Part model, mm, in its own coordinate system. A direction names the side the tool comes from. Round coordinates to 2 decimals unless told otherwise and drop trailing zeros. Order: outer loops, then holes, each group sorted by start corner. A loop starts at its lowest first (then second) coordinate and runs counter-clockwise, first axis right, second up. Notation, with made-up numbers: M -33.75,20.25 L -0.75,20.25 A23 ccw -0.75,55.25 Z; hole C 63,-32 d7. An arc over 180 degrees is marked long. One line per question, with ' | ' between items.
from build123d import *

# Parameters (mm, degrees)
ESBO_O1_R                = 1.5
ESBO_O1_R_2              = 1.25
RESSALTO_EXTRUS_O1_DEPTH = 5


with BuildPart() as part:
    # Esboço1 → Ressalto-extrusão1 (new body)
    with BuildSketch(Plane(origin=(0, 0, 0), x_dir=(1, 0, 0), z_dir=(0, 1, 0))):
        with BuildLine():
            Line((65, -55), (-65, -55))
            ThreePointArc((-65, -55), (-72.071067812, -52.071067812), (-75, -45))
            Line((-75, -45), (-75, 45))
            ThreePointArc((-75, 45), (-72.071067812, 52.071067812), (-65, 55))
            Line((-65, 55), (65, 55))
            ThreePointArc((65, 55), (72.071067812, 52.071067812), (75, 45))
            Line((75, 45), (75, -45))
            ThreePointArc((75, -45), (72.071067812, -52.071067812), (65, -55))
        make_face()
        with Locations(Location((-40, -50, 0), (0, 0, 270))):
            Circle(ESBO_O1_R, mode=Mode.SUBTRACT)
        with Locations(Location((40, -50, 0), (0, 0, 270))):
            Circle(ESBO_O1_R, mode=Mode.SUBTRACT)
        with Locations(Location((40, 50, 0), (0, 0, 90))):
            Circle(ESBO_O1_R, mode=Mode.SUBTRACT)
        with Locations(Location((-40, 50, 0), (0, 0, 90))):
            Circle(ESBO_O1_R, mode=Mode.SUBTRACT)
        with Locations(Location((17.2, 19.5, 0), (0, 0, 270))):
            Circle(ESBO_O1_R_2, mode=Mode.SUBTRACT)
        with Locations(Location((17.2, -2.5, 0), (0, 0, 270))):
            Circle(ESBO_O1_R_2, mode=Mode.SUBTRACT)
        with Locations(Location((17.2, -24.5, 0), (0, 0, 270))):
            Circle(ESBO_O1_R_2, mode=Mode.SUBTRACT)
        with Locations(Location((-17.2, -24.5, 0), (0, 0, 90))):
            Circle(ESBO_O1_R_2, mode=Mode.SUBTRACT)
        with Locations(Location((-17.2, -2.5, 0), (0, 0, 90))):
            Circle(ESBO_O1_R_2, mode=Mode.SUBTRACT)
        with Locations(Location((-17.2, 19.5, 0), (0, 0, 90))):
            Circle(ESBO_O1_R_2, mode=Mode.SUBTRACT)
        with BuildLine():
            Line((14, 30), (-14, 30))
            ThreePointArc((-14, 30), (-14.707106781, 29.707106781), (-15, 29))
            Line((-15, 29), (-15, -29))
            ThreePointArc((-15, -29), (-14.707106781, -29.707106781), (-14, -30))
            Line((-14, -30), (14, -30))
            ThreePointArc((14, -30), (14.707106781, -29.707106781), (15, -29))
            Line((15, -29), (15, 29))
            ThreePointArc((15, 29), (14.707106781, 29.707106781), (14, 30))
        make_face(mode=Mode.SUBTRACT)
    extrude(amount=RESSALTO_EXTRUS_O1_DEPTH)


solid = part.part
1) Two-plate mould, pull along Z, no slides. Class faces 3 (the face through (39.1, 2.5, 48.8)), 4 (the face through (-16, 0, -1)), 5 (the face through (72.15, 2.46, 51.99)), 6 (the face through (71.99, 2.46, -52.15)): released by +Z, released by -Z, zero draft, split by the parting line, or undercut.
The answers:
face 3: undercut | face 4: zero draft | face 5: released by +Z | face 6: released by -Z
2) Drop flat-ended pins along their axis: pin 1 (2 mm diameter, centred on x = 17.2, z = -19.5, fed in from -Y) (3 decimals); pin 2 (3.5 mm diameter, centred on x = 40, z = -50, fed in from +Y). Give the stop position or say it passes through.
The answers:
pin 1: passes through | pin 2: stops at y = 5
3) Saw through at A-A (z = -10). List the corners of the cut face in (x, y).
The answers:
outline: M -75,0 L -15,0 L -15,5 L -75,5 Z; M 15,0 L 75,0 L 75,5 L 15,5 Z
4) Probe line 1 (Z direction, x = -17.2, y = 1.7); line 2 (X direction, y = 1.35, z = -19.5); line 3 (X direction, y = 1.9, z = -11). List the from-to ranges inside material, lowest first. Write a range as [from, to].
The answers:
line 1: z = [-55, -20.75], [-18.25, 1.25], [3.75, 23.25], [25.75, 55] | line 2: x = [-75, -18.45], [-15.95, -15], [15, 15.95], [18.45, 75] | line 3: x = [-75, -15], [15, 75]
5) Saw through at D-D (x = 7.5). List the corners of the cut face in (y, z).
The answers:
outline: M 0,-55 L 5,-55 L 5,-30 L 0,-30 Z; M 0,30 L 5,30 L 5,55 L 0,55 Z
6) Which spindle directions (+Z, -Z, +X, -X, +Y, -Y) get a long thin tool onto all of the face, cutting with end or side? Do faces 1 (the face through (-15, 2, 0)), 2 (the face through (75, 2, -1)). Say none if no direction does.
The answers:
face 1: +Y, -Y | face 2: +Z, -Z, +X, +Y, -Y
7) Saw through at C-C (y = 3.95). Give the number of separate pieces and of enclosed holes in the cut face, plus the area to 3 significant figures.
The answers:
separate pieces: 1 | enclosed holes: 11 | area: 14,600 mm²
8) Saw through at B-B (x = 40). List the corners of the cut face in (y, z), plus the area to 3 significant figures.
The answers:
outline: M 0,-55 L 5,-55 L 5,-51.5 L 0,-51.5 Z; M 0,-48.5 L 5,-48.5 L 5,48.5 L 0,48.5 Z; M 0,51.5 L 5,51.5 L 5,55 L 0,55 Z | area: 520 mm²
